```python
from build123d import *

# Parameters (mm, degrees)
SKETCH1_W               = 50
SKETCH1_H               = 12.499999892
BOSS_EXTRUDE1_DEPTH     = 631
SHELL1_T                = -2
SKETCH3_W               = 50
SKETCH3_H               = 25
BOSS_EXTRUDE2_DEPTH     = 250
CUT_EXTRUDE1_DEPTH      = 470.079458784
CUT_EXTRUDE1_DEPTH_BACK = 470.079458784
SKETCH4_R               = 7.5


with BuildPart() as part:
    # Sketch1 → Boss-Extrude1 (new body)
    with BuildSketch(Plane.XY):
        with Locations((8.395937674, -2.291666613)):
            Rectangle(SKETCH1_W, SKETCH1_H)
    extrude(amount=BOSS_EXTRUDE1_DEPTH)

    # Shell1
    shell1_openings = [part.faces().sort_by_distance(p)[0] for p in [
        (8.395937674, -2.291666613, 631),
        (8.395937674, -2.291666613, 0),
    ]]
    offset(amount=SHELL1_T, openings=shell1_openings, kind=Kind.INTERSECTION)

    # Sketch3 → Boss-Extrude2 (add)
    with BuildSketch(Plane(origin=(0, 0, 0), x_dir=(1, 0, 0), z_dir=(0, 1, 0))):
        with Locations((8.395937674, -248)):
            Rectangle(SKETCH3_W, SKETCH3_H)
        with Locations((8.395937674, -383)):
            Rectangle(SKETCH3_W, SKETCH3_H)
    extrude(amount=BOSS_EXTRUDE2_DEPTH)

    # Sketch4 → Cut-Extrude1 (cut, two sides: drawn at the far end of the back side and taken through both)
    with BuildSketch(Plane(origin=(0, 0, 235.5), x_dir=(-1, 0, 0), z_dir=(0, 0, -1)).offset(-CUT_EXTRUDE1_DEPTH_BACK)):
        with Locations((-8.395937674, 225)):
            Circle(SKETCH4_R)
    extrude(amount=CUT_EXTRUDE1_DEPTH + CUT_EXTRUDE1_DEPTH_BACK, mode=Mode.SUBTRACT)


solid = part.part
```
Design review of the part built by this model. Coordinates are the model's own, in mm. A direction names the side the tool comes from. Give positions to 0.01 mm unless a question says otherwise; leave off trailing zeros. Order: outer loops, then holes, each group sorted by start corner. A loop starts at its lowest first (then second) coordinate and runs counter-clockwise, first axis right, second up. Notation, with made-up numbers: (10, 64.5) -> (61, 64.5) arc R14 ccw to (61, 82.5) -> close; hole circle Ø10 at (66, -26). An arc over 180 degrees is marked (long way). Write item = value, one per line. Start each with the question number.
(1) We need section A-A on y = 39.5. Write out the cut boundary in (x, z), plus the area to 3 significant figures.
(2) Mouldability with a two-part tool opening along X and no side actions: class faces 1 (the face through (8, -8.542, 311)), 2 (the face through (-16.604, 82, 384)), 3 (the face through (33.396, 82, 247)), 4 (the face through (8, 0, 248)) as +X half, -X half, draft (parallel to the pull), parting line (faces both ways), or undercut.
(3) We need section B-B on x = 25.5. Write out the cut boundary in (y, z), plus the area to 3 significant figures.
(4) For pin 1 (15 mm diameter, centred on x = -3.5, y = 136.5, fed in from +Z); pin 2 (1 mm diameter, centred on x = 18.5, y = 1.5, fed in from -Z); pin 3 (5 mm diameter, centred on x = 13, z = 93.5, fed in from +Y); pin 4 (1.6 mm diameter, centred on x = 2.5, y = 0.5, fed in from -Z), all flat-tipped, find the tip position at first contact; note any pin that passes through.
(5) To check wall thickness, follow line 1 along Z through (x, y) = (-12.5, 57.5); line 2 along Y through (x, z) = (14, 172); line 3 along X through (y, z) = (225, 379.5). State the ranges of each line that lie inside material, in increasing order.
(6) We need section C-C on z = 205.5. Write out the cut boundary in (x, y).
(7) We need section D-D on y = 225. Write out the cut boundary in (x, z), plus the area to 3 significant figures.
(8) For faces 5 (the face through (8, 125, 260.5)), 6 (the face through (8, 125, 395.5)), 7 (the face through (8, -6.542, 311)), 8 (the face through (8, 125, 235.5)), 9 (the face through (8, 1.958, 315)), list the 3-axis set-ups (+Z, -Z, +X, -X, +Y, -Y) from which the entire face can be reached by the end or side of a thin tool; tool diameter is ignored.
Numbers:
q1.outline = (-16.6, 235.5) -> (33.4, 235.5) -> (33.4, 260.5) -> (-16.6, 260.5) -> close; (-16.6, 370.5) -> (33.4, 370.5) -> (33.4, 395.5) -> (-16.6, 395.5) -> close
q1.area = 2,500 mm^2
q2.face_1 = draft
q2.face_2 = -X half
q2.face_3 = +X half
q2.face_4 = undercut
q3.outline = (-8.54, 0) -> (-6.54, 0) -> (-6.54, 631) -> (-8.54, 631) -> close; (0, 235.5) -> (1.96, 235.5) -> (1.96, 0) -> (3.96, 0) -> (3.96, 235.5) -> (250, 235.5) -> (250, 260.5) -> (3.96, 260.5) -> (3.96, 370.5) -> (250, 370.5) -> (250, 395.5) -> (3.96, 395.5) -> (3.96, 631) -> (1.96, 631) -> (1.96, 395.5) -> (0, 395.5) -> (0, 370.5) -> (1.96, 370.5) -> (1.96, 260.5) -> (0, 260.5) -> close
q3.area = 14,900 mm^2
q4.pin_1 = 395.5
q4.pin_2 = 0
q4.pin_3 = 3.96
q4.pin_4 = 235.5
q5.line_1 = 235.5 to 260.5, 370.5 to 395.5
q5.line_2 = -8.54 to -6.54, 1.96 to 3.96
q5.line_3 = -16.6 to 0.9, 15.9 to 33.4
q6.outline = (-16.6, -8.54) -> (33.4, -8.54) -> (33.4, 3.96) -> (-16.6, 3.96) -> close; hole (-14.6, -6.54) -> (31.4, -6.54) -> (31.4, 1.96) -> (-14.6, 1.96) -> close
q7.outline = (-16.6, 235.5) -> (0.9, 235.5) -> (0.9, 260.5) -> (-16.6, 260.5) -> close; (-16.6, 370.5) -> (0.9, 370.5) -> (0.9, 395.5) -> (-16.6, 395.5) -> close; (15.9, 235.5) -> (33.4, 235.5) -> (33.4, 260.5) -> (15.9, 260.5) -> close; (15.9, 370.5) -> (33.4, 370.5) -> (33.4, 395.5) -> (15.9, 395.5) -> close
q7.area = 1,750 mm^2
q8.face_5 = +X, -X, +Y
q8.face_6 = +Z, +X, -X, +Y
q8.face_7 = +Z, -Z
q8.face_8 = -Z, +X, -X, +Y
q8.face_9 = none
